Part model, mm, in its own coordinate system. A direction names the side the tool comes from. Give positions to 0.01 mm unless a question says otherwise; leave off trailing zeros. Write each loop counter-clockwise with the first axis right and the second up, starting at its lowest first coordinate (ties: lowest second). Pieces come first, ordered by that corner, then holes. Notation, with made-up numbers: M 0,-12.75 L 43,-12.75 A10 ccw 43,-0.75 Z; hole C 57.25,75 d10. An arc over 180 degrees is marked long. Use a Markdown table: item, result.
Autodesk Inventor part; units mm, degrees
ref_plane "YZ Plane" through (0, 0, 0) normal (1, 0, 0) x (0, 1, 0)
ref_plane "XZ Plane" through (0, 0, 0) normal (0, 1, 0) x (-1, 0, 0)
ref_plane "XY Plane" through (0, 0, 0) normal (0, 0, 1) x (1, 0, 0)
sketch "Sketch1" plane through (0, 0, 0) normal (0, 1, 0) x (-1, 0, 0)
  line L0 (63.5, -48.133) -> (79.8363, -48.133)
  line L1 (46.2829, -48.133) -> (63.5, -48.133)
  line L2 (43.9969, -84.201) -> (43.9969, -50.419)
  line L3 (63.5, -86.487) -> (46.2829, -86.487)
  line L4 (79.8363, -86.487) -> (63.5, -86.487)
  line L5 (82.1223, -50.419) -> (82.1223, -84.201)
  arc A0 (79.8363, -86.487) -> (82.1223, -84.201) centre (79.8363, -84.201) ccw
  arc A1 (82.1223, -50.419) -> (79.8363, -48.133) centre (79.8363, -50.419) ccw
  arc A2 (46.2829, -48.133) -> (43.9969, -50.419) centre (46.2829, -50.419) ccw
  arc A3 (43.9969, -84.201) -> (46.2829, -86.487) centre (46.2829, -84.201) ccw
  line L6 (63.5, -89.987) -> (46.2829, -89.987)
  arc A4 (40.4969, -84.201) -> (46.2829, -89.987) centre (46.2829, -84.201) ccw
  line L7 (40.4969, -84.201) -> (40.4969, -50.419)
  arc A5 (46.2829, -44.633) -> (40.4969, -50.419) centre (46.2829, -50.419) ccw
  line L8 (46.2829, -44.633) -> (63.5, -44.633)
  line L9 (63.5, -44.633) -> (79.8363, -44.633)
  arc A6 (85.6223, -50.419) -> (79.8363, -44.633) centre (79.8363, -50.419) ccw
  line L10 (85.6223, -50.419) -> (85.6223, -84.201)
  arc A7 (79.8363, -89.987) -> (85.6223, -84.201) centre (79.8363, -84.201) ccw
  line L11 (79.8363, -89.987) -> (63.5, -89.987)
  dimension "d4" = 3.5
extrude "Extrusion1" add sketch "Sketch1" along normal blind 2 contours L0 A1 L5 A0 L4 L3 A3 L2 A2 L1 | L6 A4 L7 A5 L8 L9 A6 L10 A7 L11
sketch "Sketch3" plane through (0, 2, 0) normal (0, 1, 0) x (1, 0, 0)
  line L0 (-82.1223, 50.419) -> (-82.1223, 84.201)
  arc A0 (-82.1223, 50.419) -> (-79.8363, 48.133) centre (-79.8363, 50.419) ccw
  line L1 (-63.5, 48.133) -> (-79.8363, 48.133)
  line L2 (-46.2829, 48.133) -> (-63.5, 48.133)
  arc A1 (-46.2829, 48.133) -> (-43.9969, 50.419) centre (-46.2829, 50.419) ccw
  line L3 (-43.9969, 84.201) -> (-43.9969, 50.419)
  arc A2 (-43.9969, 84.201) -> (-46.2829, 86.487) centre (-46.2829, 84.201) ccw
  line L4 (-63.5, 86.487) -> (-46.2829, 86.487)
  line L5 (-79.8363, 86.487) -> (-63.5, 86.487)
  arc A3 (-79.8363, 86.487) -> (-82.1223, 84.201) centre (-79.8363, 84.201) ccw
  line L6 (-63.5, 86.287) -> (-46.2829, 86.287)
  arc A4 (-44.1969, 84.201) -> (-46.2829, 86.287) centre (-46.2829, 84.201) ccw
  line L7 (-44.1969, 84.201) -> (-44.1969, 50.419)
  arc A5 (-46.2829, 48.333) -> (-44.1969, 50.419) centre (-46.2829, 50.419) ccw
  line L8 (-46.2829, 48.333) -> (-63.5, 48.333)
  line L9 (-63.5, 48.333) -> (-79.8363, 48.333)
  arc A6 (-81.9223, 50.419) -> (-79.8363, 48.333) centre (-79.8363, 50.419) ccw
  line L10 (-81.9223, 50.419) -> (-81.9223, 84.201)
  arc A7 (-79.8363, 86.287) -> (-81.9223, 84.201) centre (-79.8363, 84.201) ccw
  line L11 (-79.8363, 86.287) -> (-63.5, 86.287)
  dimension "d7" = 0.2
extrude "Extrusion3" add sketch "Sketch3" along normal blind 4.484 contours L6 A4 L7 A5 L8 L9 A6 L10 A7 L11
properties part number "Plug"
1. Cut at A-A, the plane z = -81. Give the cut face in (x, y), then the cut area to 3 significant figures.
Findings below:
| item | result |
|---|---|
| outline | M -85.62,0 L -40.5,0 L -40.5,2 L -44.2,2 L -44.2,6.48 L -81.92,6.48 L -81.92,2 L -85.62,2 Z |
| area | 259 mm2 |
2. Drill centre lines: L1, parallel to Z at x = -63, y = 2.5; L2, parallel to X at y = 3.5, z = -75; L3, parallel to Y at x = -56, z = -46.5. Where is each one in solid material? Low to high.
Findings below:
| item | result |
|---|---|
| L1 | -86.29 to -48.33 |
| L2 | -81.92 to -44.2 |
| L3 | 0 to 2 |
3. Drop flat-ended pins along their axis: P1, Ø3, axis at x = -49.5, y = 4.5, coming from the +Z side; P2, Ø2, axis at y = 4.5, z = -66.5, coming from the -X side; P3, Ø1.3, axis at y = 4, z = -71, coming from the +X side; P4, Ø2, axis at y = 2.5, z = -65.5, coming from the -X side. Give the stop position or say it passes through.
Findings below:
| item | result |
|---|---|
| P1 | z = -48.33 |
| P2 | x = -81.92 |
| P3 | x = -44.2 |
| P4 | x = -85.62 |
4. Tool access for faces 1 (the flat face through (-43, 2, -67)), 2 (the cylindrical face through (-44.82, 4.21, -85.69)), 3 (the cylindrical face through (-81.327, 4.211, -85.66)), 4 (the cylindrical face through (-81.3, 4.21, -48.93)): list every direction of +Z, -Z, +X, -X, +Y, -Y with a clear straight run to the whole face (end or side of a thin tool).
Findings below:
| item | result |
|---|---|
| face 1 | +Y |
| face 2 | -Z, +X, +Y |
| face 3 | -Z, -X, +Y |
| face 4 | +Z, -X, +Y |
5. Cut at B-B, the plane y = 3.5. Give the cut face in (x, z).
Findings below:
| item | result |
|---|---|
| outline | M -81.92,-84.2 A2.09 ccw -79.84,-86.29 L -46.28,-86.29 A2.09 ccw -44.2,-84.2 L -44.2,-50.42 A2.09 ccw -46.28,-48.33 L -79.84,-48.33 A2.09 ccw -81.92,-50.42 Z |
